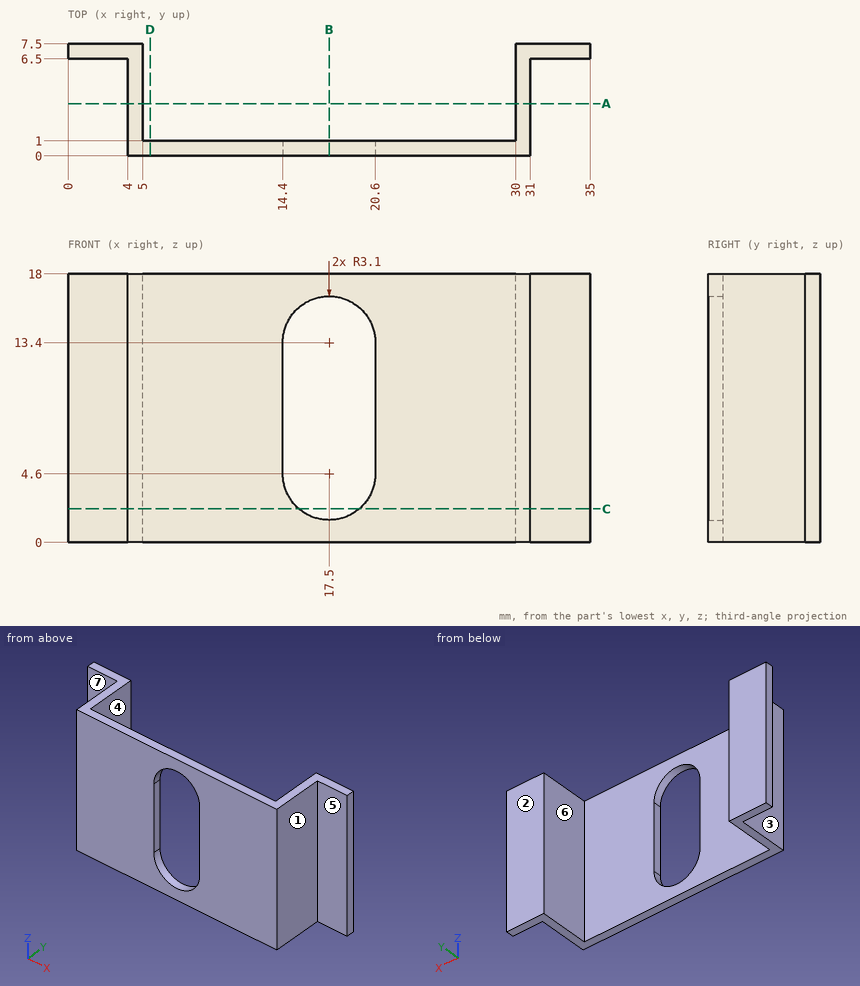
Geometry check sheet. Reference: drawing and pictorial views, mm from the part's lowest x, y, z. A direction names the side the tool comes from. Give positions to 0.01 mm unless a question says otherwise; leave off trailing zeros. Loops run counter-clockwise (first coordinate to the right, second up) from the corner with the lowest first, then second, coordinate; pieces in that order, holes last. Notation, with made-up numbers: M 9,88 L 53,88 A16 ccw 53,103 Z; hole C -27.75,43 d9. An arc over 180 degrees is marked long. One line per question, with ' | ' between items.
Item 1: Tool access check on the marked faces 5, 6 and 7. Record the directions out of +Z, -Z, +X, -X, +Y, -Y that give a thin tool (end or side, any length) a straight path to the whole face; none if there is none.
Completed:
face 5: +Z, -Z, +X, -Y | face 6: +Z, -Z, +Y | face 7: +Z, -Z, -X, -Y
Item 2: Thickness scan on line 1 (X direction, y = 1.75, z = 8); line 2 (Y direction, x = 20, z = 15.5); line 3 (X direction, y = 7, z = 12.5). Record the ranges inside material, lowest first. Write a range as [from, to].
Completed:
line 1: x = [4, 5], [30, 31] | line 2: y = [0, 1] | line 3: x = [0, 5], [30, 35]
Item 3: Section check C-C, the plane z = 2.25. Record the cut outline in (x, y), plus the area to 3 significant figures.
Completed:
outline: M 0,6.5 L 4,6.5 L 4,0 L 15.48,0 L 15.48,1 L 5,1 L 5,7.5 L 0,7.5 Z; M 19.52,0 L 31,0 L 31,6.5 L 35,6.5 L 35,7.5 L 30,7.5 L 30,1 L 19.52,1 Z | area: 44.0 mm^2
Item 4: Section check B-B, the plane x = 17.5. Record the cut outline in (y, z), plus the area to 3 significant figures.
Completed:
outline: M 0,0 L 1,0 L 1,1.5 L 0,1.5 Z; M 0,16.5 L 1,16.5 L 1,18 L 0,18 Z | area: 3.00 mm^2
Item 5: Draft check along X on the marked faces 1, 2, 3 and 4. Enter one of: +X half, -X half, draft (parallel to the pull), parting line (faces both ways), or undercut.
Completed:
face 1: +X half | face 2: draft | face 3: -X half | face 4: undercut
Item 6: Section check D-D, the plane x = 5.5. Record the cut outline in (y, z), plus the area to 3 significant figures.
Completed:
outline: M 0,0 L 1,0 L 1,18 L 0,18 Z | area: 18.0 mm^2
Item 7: Depth check by flat-ended pin: P1, Ø2, axis at x = 8, z = 7, coming from the +Y side; P2, Ø3, axis at y = 4.5, z = 10, coming from the -X side; P3, Ø2, axis at y = 2.5, z = 12.5, coming from the +X side. Enter the tip coordinate at first touch or a pass-through.
Completed:
P1: stops at y = 1 | P2: stops at x = 4 | P3: stops at x = 31
Item 8: Section check A-A, the plane y = 3.5. Record the cut outline in (x, z).
Completed:
outline: M 4,0 L 5,0 L 5,18 L 4,18 Z; M 30,0 L 31,0 L 31,18 L 30,18 Z
